The model under review builds one solid part; all positions refer to its coordinate system, in mm. Face numbers are marked on the shaded views. A direction names the side the tool comes from. Round coordinates to 2 decimals unless told otherwise and drop trailing zeros. Write each loop counter-clockwise with the first axis right and the second up, starting at its lowest first coordinate (ties: lowest second). Pieces come first, ordered by that corner, then holes. Notation, with made-up numbers: (-15, 50) -> (24, 50) arc R22 ccw to (24, 70) -> close; hole circle Ø10 at (24, 71). An arc over 180 degrees is marked (long way). Use CSV: the item, a comma, the result in double quotes. Start each with the question number.
1) Take a section at B-B, the plane y = 21. Give the boundary of the cut face in (x, z).
2) For pin 1 Ø0.9 at (y, z) = (-4, 0) entering from +X (3 decimals); pin 2 Ø5 at (x, y) = (3, 14.5) entering from +Z; pin 3 Ø1 at (x, z) = (5, 12) entering from +Y; pin 4 Ø13 at (x, z) = (6.5, 2.5) entering from +Y, all flat-tipped, find the tip position at first contact; note any pin that passes through.
3) Wall thickness on probe 1 along X at (y, z) = (11.5, -6.5); probe 2 along Y at (x, z) = (7.25, -11); probe 3 along Z at (x, y) = (3, 12): over which ranges is each line inside the solid? List them lowest first. Write a range as [from, to].
4) Take a section at A-A, the plane y = 4. Give the boundary of the cut face in (x, z).
5) Mouldability with a two-part tool opening along Z and no side actions: class the marked faces 1, 2, 3 and 4 as released by +Z, released by -Z, zero draft, split by the parting line, or undercut.
6) Machinability: for the marked faces 5, 6, 7, 8 and 9, which of the approach directions +Z, -Z, +X, -X, +Y, -Y give a long, thin tool a straight path to every point of the face, cutting with its end or side? Answer none if there is none.
Autodesk Inventor part; units mm, degrees
ref_plane "Work Plane1" through (6.9, 0, 13.6) normal (1, 0, 0) x (0, 0, -1)
ref_plane "YZ Plane" through (0, 0, 0) normal (1, 0, 0) x (0, 1, 0)
ref_plane "XZ Plane" through (0, 0, 0) normal (0, 1, 0) x (-1, 0, 0)
sketch "Sketch1" plane through (0, 0, 0) normal (0, 1, 0) x (-1, 0, 0)
  line L0 (8.9, 17.6) -> (-8.9, 17.6)
  line L1 (-8.9, 17.6) -> (-8.9, -17.6)
  line L2 (-8.9, -17.6) -> (8.9, -17.6)
  line L3 (8.9, -17.6) -> (8.9, 17.6)
  point P0 (0, 0)
  point P1 (8.9, 0)
  point P2 (0, -17.6)
  dimension "d0" = 35.2
  dimension "d1" = 17.8
extrude "Extrusion1" add sketch "Sketch1" along normal blind 16
sketch "Sketch2" plane through (0, 16, 0) normal (0, 1, 0) x (1, 0, 0)
  ellipse E0 centre (0, 0) end of major axis (0, 21) minor radius 13
  dimension "d4" = 21
  dimension "d5" = 13
extrude "Extrusion2" add sketch "Sketch2" along normal blind 3
fillet "Fillet1" radius 4 4 edges at (8.9, 8, 17.6) (8.9, 8, -17.6) (-8.9, 8, 17.6) (-8.9, 8, -17.6)
ref_plane "Work Plane1" through (6.9, 0, 13.6) normal (1, 0, 0) x (0, 0, -1)
sketch "Sketch3" plane through (6.9, 0, 13.6) normal (1, 0, 0) x (0, 0, -1)
  line L0 (34.6, 19) -> (-7.4, 19)
  line L1 (27.6, 19) -> (6.5786, 24)
  line L2 (6.5786, 24) -> (-0.4, 19)
  line L3 (-0.4, 19) -> (27.6, 19)
  point P0 (13.6, 0)
  dimension "d10" = 7
  dimension "d11" = 7
  dimension "d12" = 5
  dimension "d13" = 131
extrude "Extrusion3" add sketch "Sketch3" against normal blind 13.8
sketch "Sketch4" plane through (0, 0, 0) normal (0, -1, 0) x (1, 0, 0)
  line L0 (3.175, 11.1) -> (-3.175, 11.1)
  line L1 (-3.175, 11.1) -> (-3.175, 10.3)
  line L2 (-3.175, 10.3) -> (3.175, 10.3)
  line L3 (3.175, 10.3) -> (3.175, 11.1)
  line L4 (3.175, 0.4) -> (-3.175, 0.4)
  line L5 (-3.175, 0.4) -> (-3.175, -0.4)
  line L6 (-3.175, -0.4) -> (3.175, -0.4)
  line L7 (3.175, -0.4) -> (3.175, 0.4)
  line L8 (3.175, -10.3) -> (-3.175, -10.3)
  line L9 (-3.175, -10.3) -> (-3.175, -11.1)
  line L10 (-3.175, -11.1) -> (3.175, -11.1)
  line L11 (3.175, -11.1) -> (3.175, -10.3)
  line L12 (0, 10.3) -> (0, 0.4)
  line L13 (0, -0.4) -> (0, -10.3)
  line L14 (0, -11.1) -> (0, -21)
  ellipse E0 centre (0, 0) end of major axis (0, 21) minor radius 13
  line L15 (0, 11.1) -> (0, 21)
  point P0 (3.175, 0)
  dimension "d16" = 0.8
  dimension "d17" = 6.35
extrude "Extrusion4" add sketch "Sketch4" along normal blind 8.5 contours L3 L2 L1 L0 | L4 L7 L6 L5 | L10 L9 L8 L11
properties part number "SwitchRocker"
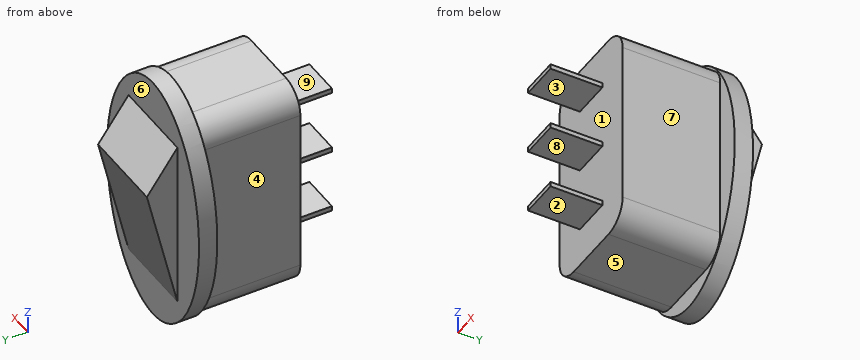
Values found:
1,outline,"(-6.9, -5.59) -> (6.9, -5.59) -> (6.9, 11.21) -> (-6.9, 11.21) -> close"
2,pin 1,"x = 3.175"
2,pin 2,"z = 20.94"
2,pin 3,"y = 20.79"
2,pin 4,"y = 24"
3,probe 1,"[-8.9, 8.9]"
3,probe 2,"[0, 19]"
3,probe 3,"[-17.6, 17.6]"
4,outline,"(-8.9, -13.6) arc R4 ccw to (-4.9, -17.6) -> (4.9, -17.6) arc R4 ccw to (8.9, -13.6) -> (8.9, 13.6) arc R4 ccw to (4.9, 17.6) -> (-4.9, 17.6) arc R4 ccw to (-8.9, 13.6) -> close"
5,face 1,"undercut"
5,face 2,"released by -Z"
5,face 3,"undercut"
5,face 4,"zero draft"
6,face 5,"-Z, +X, -X, -Y"
6,face 6,"+Y"
6,face 7,"+Z, -Z, +X, -Y"
6,face 8,"+X, -X, -Y"
6,face 9,"+Z, +X, -X, -Y"
